from build123d import *

# Parameters (mm, degrees)
P_DORYS_W                                         = 120
P_DORYS_H                                         = 100
P_IDAT_VYSUNUT_M1_DEPTH                           = 2
ZAOBLIT1_R                                        = 2
SKICA2_W                                          = 114.8
SKICA2_H                                          = 94.8
SKICA2_W_2                                        = 109.8
SKICA2_H_2                                        = 89.8
SKICA2_W_3                                        = 4
SKICA2_H_3                                        = 7
SKICA2_H_4                                        = 3.5
P_IDAT_VYSUNUT_M2_DEPTH                           = 2
P_IDAT_VYSUNUT_M3_DEPTH                           = 6
V_LCOV_ZAHLOUBEN_PRO_M6_ROUBY_S_V_LCO_D           = 3.4
V_LCOV_ZAHLOUBEN_PRO_M6_ROUBY_S_V_LCO_DEPTH       = 9.1
V_LCOV_ZAHLOUBEN_PRO_M6_ROUBY_S_V_LCO_CBORE_D     = 3.9
V_LCOV_ZAHLOUBEN_PRO_M6_ROUBY_S_V_LCO_CBORE_DEPTH = 4
SKICA7_R                                          = 2.25
ODEBRAT_VYSUNUT_M1_DEPTH                          = 6


with BuildPart() as part:
    # půdorys → Přidat vysunutím1 (new body)
    with BuildSketch(Plane.XY):
        Rectangle(P_DORYS_W, P_DORYS_H)
    extrude(amount=P_IDAT_VYSUNUT_M1_DEPTH)

    # Zaoblit1
    zaoblit1_edges = [part.edges().sort_by_distance(p)[0] for p in [
        (60, -50, 1),
        (-60, -50, 1),
        (-60, 50, 1),
        (60, 50, 1),
    ]]
    fillet(zaoblit1_edges, radius=ZAOBLIT1_R)

    # Skica2 → Přidat vysunutím2 (add)
    # profile 1 of 4: a face of its own
    with BuildSketch(Plane.XY.offset(2)):
        Rectangle(SKICA2_W, SKICA2_H)
        Rectangle(SKICA2_W_2, SKICA2_H_2, mode=Mode.SUBTRACT)
    # profile 2 of 4: a face of its own
    with BuildSketch(Plane.XY.offset(2)):
        with Locations((52.9, 0)):
            Rectangle(SKICA2_W_3, SKICA2_H_3)
    # profile 3 of 4: a face of its own
    with BuildSketch(Plane.XY.offset(2)):
        with Locations((-52.9, -1.75)):
            Rectangle(SKICA2_W_3, SKICA2_H_4)
    # profile 4 of 4: a face of its own
    with BuildSketch(Plane.XY.offset(2)):
        with Locations((-52.9, 1.75)):
            Rectangle(SKICA2_W_3, SKICA2_H_4)
    extrude(amount=P_IDAT_VYSUNUT_M2_DEPTH)

    # Skica3 → Přidat vysunutím3 (add)
    with BuildSketch(Plane.XY.offset(4)):
        Polygon((54.9, -47.4), (57.4, -47.4), (57.4, 47.4), (54.9, 47.4), (54.9, 44.9), (54.9, 3.5), (50.9, 3.5), (50.9, -3.5), (54.9, -3.5), (54.9, -44.9), align=None)
        Polygon((-57.4, -47.4), (-54.9, -47.4), (-54.9, -44.9), (-54.9, -3.5), (-50.9, -3.5), (-50.9, 3.5), (-54.9, 3.5), (-54.9, 44.9), (-54.9, 47.4), (-57.4, 47.4), align=None)
    extrude(amount=P_IDAT_VYSUNUT_M3_DEPTH)

    # Válcové zahloubení pro M6 šrouby s válcovou hlavou zaoblenou1
    with Locations(Plane(origin=(-50.9, 0, 6), x_dir=(0, 0, 1), z_dir=(1, 0, 0))):
        with Locations((0, 0)):
            v_lcov_zahlouben_pro_m6_rouby_s_v_lco = CounterBoreHole(V_LCOV_ZAHLOUBEN_PRO_M6_ROUBY_S_V_LCO_D / 2, V_LCOV_ZAHLOUBEN_PRO_M6_ROUBY_S_V_LCO_CBORE_D / 2, V_LCOV_ZAHLOUBEN_PRO_M6_ROUBY_S_V_LCO_CBORE_DEPTH, depth=V_LCOV_ZAHLOUBEN_PRO_M6_ROUBY_S_V_LCO_DEPTH)

    # Zrcadlit1: Válcové zahloubení pro M6 šrouby s válcovou hlavou zaoblenou1 across plane
    add(v_lcov_zahlouben_pro_m6_rouby_s_v_lco.mirror(Plane(origin=(0, 0, 0), x_dir=(0, 0, 1), z_dir=(1, 0, 0))), mode=Mode.SUBTRACT)

    # Skica7 → Odebrat vysunutím1 (cut)
    with BuildSketch(Plane(origin=(0, 0, 0), x_dir=(-1, 0, 0), z_dir=(0, 0, -1))):
        with BuildLine():
            ThreePointArc((37.290080195, 9.875934852), (41, 2.4173e-05), (37.290112025, -9.875898463))
            Line((37.290112025, -9.875898463), (40.123514646, -12.709301084))
            ThreePointArc((40.123514646, -12.709301084), (45, 2.4153e-05), (40.123482334, 12.709336991))
            Line((40.123482334, 12.709336991), (37.290080195, 9.875934852))
        make_face()
        with BuildLine():
            ThreePointArc((35.872258171, -8.458044609), (39, 2.4191e-05), (35.872226693, 8.45808135))
            Line((35.872226693, 8.45808135), (33.031631805, 5.617486462))
            ThreePointArc((33.031631805, 5.617486462), (35, 2.427e-05), (33.031662102, -5.617448539))
            Line((33.031662102, -5.617448539), (35.872258171, -8.458044609))
        make_face()
        with Locations((42, -16)):
            Circle(SKICA7_R)
        with Locations((42, 16)):
            Circle(SKICA7_R)
        with BuildLine():
            ThreePointArc((16.124101537, 11.290112025), (26, 15), (35.875898463, 11.290112025))
            Line((35.875898463, 11.290112025), (38.709301084, 14.123514646))
            ThreePointArc((38.709301084, 14.123514646), (26, 19), (13.290698916, 14.123514646))
            Line((13.290698916, 14.123514646), (16.124101537, 11.290112025))
        make_face()
        with BuildLine():
            Line((38.709301084, -14.123514646), (35.875898463, -11.290112025))
            ThreePointArc((35.875898463, -11.290112025), (25.999975827, -15), (16.124065148, -11.290080195))
            Line((16.124065148, -11.290080195), (13.290663009, -14.123482334))
            ThreePointArc((13.290663009, -14.123482334), (25.999975847, -19), (38.709301084, -14.123514646))
        make_face()
        with BuildLine():
            Line((31.617448539, 7.031662102), (34.458044609, 9.872258171))
            ThreePointArc((34.458044609, 9.872258171), (26, 13), (17.541955391, 9.872258171))
            Line((17.541955391, 9.872258171), (20.382551461, 7.031662102))
            ThreePointArc((20.382551461, 7.031662102), (26, 9), (31.617448539, 7.031662102))
        make_face()
        with BuildLine():
            ThreePointArc((17.54191865, -9.872226693), (25.999975809, -13), (34.458044609, -9.872258171))
            Line((34.458044609, -9.872258171), (31.617448539, -7.031662102))
            ThreePointArc((31.617448539, -7.031662102), (25.99997573, -9), (20.382513538, -7.031631805))
            Line((20.382513538, -7.031631805), (17.54191865, -9.872226693))
        make_face()
        with BuildLine():
            ThreePointArc((18.968337898, -5.617448539), (17, 0), (18.968337898, 5.617448539))
            Line((18.968337898, 5.617448539), (16.127741829, 8.458044609))
            ThreePointArc((16.127741829, 8.458044609), (13, 0), (16.127741829, -8.458044609))
            Line((16.127741829, -8.458044609), (18.968337898, -5.617448539))
        make_face()
        with Locations((10, 16)):
            Circle(SKICA7_R)
        with BuildLine():
            Line((14.709887975, 9.875898463), (11.876485354, 12.709301084))
            ThreePointArc((11.876485354, 12.709301084), (7, 0), (11.876485354, -12.709301084))
            Line((11.876485354, -12.709301084), (14.709887975, -9.875898463))
            ThreePointArc((14.709887975, -9.875898463), (11, 0), (14.709887975, 9.875898463))
        make_face()
        with Locations((10, -16)):
            Circle(SKICA7_R)
    extrude(amount=-ODEBRAT_VYSUNUT_M1_DEPTH, mode=Mode.SUBTRACT)


solid = part.part
Design review of the part built by this model. Coordinates are the model's own, in mm. A direction names the side the tool comes from. Give positions to 0.01 mm unless a question says otherwise; leave off trailing zeros. Loops run counter-clockwise (first coordinate to the right, second up) from the corner with the lowest first, then second, coordinate; pieces in that order, holes last. Notation, with made-up numbers: M -13,51.5 L 18,51.5 A12 ccw 18,62.5 Z; hole C 62,51.5 d2. An arc over 180 degrees is marked long. Answer as a JSON object with one key per item and string values.
Item 1: We need section C-C (x = 42). State the section outline as (y, z) points.
Output values:
{"outline": "M -50,0 L 50,0 L 50,2 L 47.4,2 L 47.4,4 L 44.9,4 L 44.9,2 L -44.9,2 L -44.9,4 L -47.4,4 L -47.4,2 L -50,2 Z"}
Item 2: Machinability: for faces 1 (the face through (54.9, -25, 6)), 2 (the face through (-37.273, 12.687, 0.986)), 3 (the face through (-1, 1, 0)), which of the approach directions +Z, -Z, +X, -X, +Y, -Y give a long, thin tool a straight path to every point of the face, cutting with its end or side? Answer none if there is none.
Output values:
{"face 1": "+Z", "face 2": "+Z, -Z", "face 3": "-Z, +X, -X, +Y, -Y"}
Item 3: We need section B-B (x = -53). State the section outline as (y, z) points, and give its area (3 significant figures).
Output values:
{"outline": "M -50,0 L 50,0 L 50,2 L 47.4,2 L 47.4,4 L 44.9,4 L 44.9,2 L 3.5,2 L 3.5,10 L -3.5,10 L -3.5,2 L -44.9,2 L -44.9,4 L -47.4,4 L -47.4,2 L -50,2 Z; hole C 0,6 d3.9", "area": "254 mm2"}
Item 4: We need section A-A (z = 6). Count the separate pieces of the cut face and the enclosed holes in it, and give its area (3 significant figures).
Output values:
{"separate pieces": "4", "enclosed holes": "0", "area": "482 mm2"}
Item 5: For P1, Ø1.5, axis at x = 44.5, y = -16.5, coming from the -Z side; P2, Ø2.5, axis at y = 6, z = 7, coming from the -X side; P3, Ø2, axis at y = -32, z = 5.5, coming from the +X side; P4, Ø6, axis at x = 27, y = 16, coming from the +Z side, all flat-tipped, find the tip position at first contact; note any pin that passes through.
Output values:
{"P1": "stops at z = 0", "P2": "stops at x = -57.4", "P3": "stops at x = 57.4", "P4": "stops at z = 2"}
Item 6: Wall thickness on line 1 along Y through (x, z) = (53.2, 6); line 2 along X through (y, z) = (-11, 9.5); line 3 along Y through (x, z) = (21.5, 2.25): over which ranges is each line inside the solid? List them lowest first.
Output values:
{"line 1": "y = -3.5 to -1.95, 1.95 to 3.5", "line 2": "x = -57.4 to -54.9, 54.9 to 57.4", "line 3": "y = -47.4 to -44.9, 44.9 to 47.4"}
Item 7: Mouldability with a two-part tool opening along X and no side actions: class faces 4 (the face through (0.3, 47.4, 3.6)), 5 (the face through (57.4, -1, 4)), 6 (the face through (-33.018, 8.432, 0.986)) as pulls with the +X half, pulls with the -X half, needs draft (parallel to the pull), parting line crosses it, or undercut.
Output values:
{"face 4": "needs draft", "face 5": "pulls with the +X half", "face 6": "undercut"}
Item 8: We need section D-D (y = 27). State the section outline as (x, z) points.
Output values:
{"outline": "M -60,0 L 60,0 L 60,2 L 57.4,2 L 57.4,10 L 54.9,10 L 54.9,2 L -54.9,2 L -54.9,10 L -57.4,10 L -57.4,2 L -60,2 Z"}
